```python
from build123d import *

# Parameters (mm, degrees)
BOSS_EXTRUDE1_DEPTH = 5
SKETCH11_R          = 7.25
BOSS_EXTRUDE3_DEPTH = 0.5
SKETCH12_R          = 6
BOSS_EXTRUDE4_DEPTH = 3.5
SKETCH13_R          = 1.55
CUT_EXTRUDE1_DEPTH  = 20.5
CUT_EXTRUDE2_DEPTH  = 2.6
SKETCH17_R          = 1.55
CUT_EXTRUDE4_DEPTH  = 10.02
SKETCH18_R          = 2.85
CUT_EXTRUDE5_DEPTH  = 2.85
CUT_EXTRUDE7_DEPTH  = 10


with BuildPart() as part:
    # Sketch2 → Boss-Extrude1 (new body)
    with BuildSketch(Plane.XY):
        with BuildLine():
            Line((0, 11.5), (90, 11.5))
            ThreePointArc((90, 11.5), (101.5, 0), (90, -11.5))
            Line((90, -11.5), (0, -11.5))
            ThreePointArc((0, -11.5), (-11.5, 0), (0, 11.5))
        make_face()
    extrude(amount=-BOSS_EXTRUDE1_DEPTH)

    # Sketch11 → Boss-Extrude3 (add)
    with BuildSketch(Plane.XY):
        with Locations((90, 0)):
            Circle(SKETCH11_R)
    extrude(amount=BOSS_EXTRUDE3_DEPTH)

    # Sketch12 → Boss-Extrude4 (add)
    with BuildSketch(Plane.XY.offset(0.5)):
        with Locations((90, 0)):
            Circle(SKETCH12_R)
    extrude(amount=BOSS_EXTRUDE4_DEPTH)

    # Sketch13 → Cut-Extrude1 (cut)
    with BuildSketch(Plane.XY.offset(4)):
        with Locations((90, 0)):
            Circle(SKETCH13_R)
    extrude(amount=-CUT_EXTRUDE1_DEPTH, mode=Mode.SUBTRACT)

    # Sketch14 → Cut-Extrude2 (cut)
    with BuildSketch(Plane(origin=(0, 0, -5), x_dir=(-1, 0, 0), z_dir=(0, 0, -1))):
        Polygon((-93.213605432, -0.355068252), (-91.299304589, -2.960598068), (-88.085699158, -2.605529815), (-86.786394568, 0.355068252), (-88.700695411, 2.960598068), (-91.914300842, 2.605529815), align=None)
    extrude(amount=-CUT_EXTRUDE2_DEPTH, mode=Mode.SUBTRACT)

    # Sketch17 → Cut-Extrude4 (cut)
    with BuildSketch(Plane.XY):
        with Locations((0, 7)):
            Circle(SKETCH17_R)
        with Locations((0, -7)):
            Circle(SKETCH17_R)
        with Locations((-7, 0)):
            Circle(SKETCH17_R)
        with Locations((7, 0)):
            Circle(SKETCH17_R)
    extrude(amount=-CUT_EXTRUDE4_DEPTH, mode=Mode.SUBTRACT)

    # Sketch18 → Cut-Extrude5 (cut)
    with BuildSketch(Plane.XY):
        Circle(SKETCH18_R)
    extrude(amount=-CUT_EXTRUDE5_DEPTH, mode=Mode.SUBTRACT)

    # Sketch19 → Cut-Extrude7 (cut)
    with BuildSketch(Plane.XY):
        with BuildLine():
            Line((30.521520475, -8), (15.521520475, 8))
            ThreePointArc((15.521520475, 8), (12.69309335, 6.828427125), (11.521520475, 4))
            Line((11.521520475, 4), (11.521520475, -4))
            ThreePointArc((11.521520475, -4), (12.69309335, -6.828427125), (15.521520475, -8))
            Line((15.521520475, -8), (30.521520475, -8))
        make_face()
        Polygon((50.521520475, 8), (20.521520475, 8), (35.521520475, -8), align=None)
        Polygon((70.521520475, -8), (55.521520475, 8), (40.521520475, -8), align=None)
        with BuildLine():
            Line((75.521520475, 8), (60.521520475, 8))
            Line((60.521520475, 8), (75.521520475, -8))
            ThreePointArc((75.521520475, -8), (78.3499476, -6.828427125), (79.521520475, -4))
            Line((79.521520475, -4), (79.521520475, 4))
            ThreePointArc((79.521520475, 4), (78.3499476, 6.828427125), (75.521520475, 8))
        make_face()
    extrude(amount=-CUT_EXTRUDE7_DEPTH, mode=Mode.SUBTRACT)


solid = part.part
```
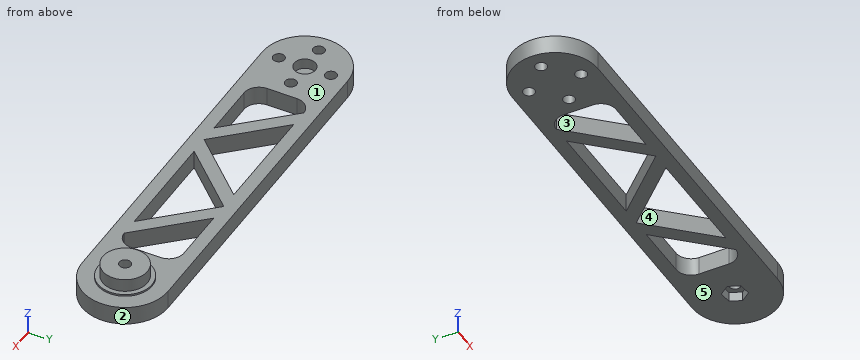
Geometry check sheet. Reference: the model listing, model coordinates, mm. Face numbers are marked on the shaded views. A direction names the side the tool comes from. Coordinates: 2 decimals unless noted, no trailing zeros. Write each loop counter-clockwise with the first axis right and the second up, starting at its lowest first coordinate (ties: lowest second). Pieces come first, ordered by that corner, then holes. Notation, with made-up numbers: (24, -15.5) -> (65, -15.5) arc R26 cw to (65, 7.5) -> close; hole circle Ø11 at (60, 70). An arc over 180 degrees is marked (long way). Use CSV: the item, a comma, the result in double quotes. Start each with the question number.
Item 1: Depth check by flat-ended pin: pin 1 Ø1.5 at (y, z) = (1, -1.5) entering from -X; pin 2 Ø4 at (x, y) = (9.5, -4.5) entering from +Z; pin 3 Ø5 at (y, z) = (-6, -1) entering from +X; pin 4 Ø6.5 at (x, y) = (91, 1) entering from -Z. Enter the tip coordinate at first touch or a pass-through.
Item 2: Cross-section at A-A, the plane x = 7. Record the cut outline in (y, z).
Item 3: Thickness scan on line 1 (Y direction, x = 0, z = -3.55); line 2 (X direction, y = -6, z = -3.75); line 3 (X direction, y = 3, z = -3.5). Record the ranges inside material, lowest first.
Item 4: Cross-section at B-B, the plane z = 1.75. Record the cut outline in (x, y).
Item 5: Set-up check for the marked faces 4 and 5: record each of +Z, -Z, +X, -X, +Y, -Y from which the full face is reachable in a straight line by a thin tool's end or side.
Item 6: Mould release check, pull along X, two halves, no side actions. Record for the marked faces 1, 2 and 3: released by +X, released by -X, zero draft, split by the parting line, or undercut.
Item 7: Cross-section at C-C, the plane x = -7. Record the cut outline in (y, z), plus the area to 3 significant figures.
Answers:
1,pin 1,"x = -11.5"
1,pin 2,"z = 0"
1,pin 3,"x = 100.95"
1,pin 4,"z = -5"
2,outline,"(-11.5, -5) -> (-1.55, -5) -> (-1.55, 0) -> (-11.5, 0) -> close; (1.55, -5) -> (11.5, -5) -> (11.5, 0) -> (1.55, 0) -> close"
3,line 1,"-11.5 to -8.55, -5.45 to 5.45, 8.55 to 11.5"
3,line 2,"-9.81 to -1.18, 1.18 to 12.06, 28.65 to 33.65, 37.4 to 42.4, 68.65 to 73.65, 78.99 to 99.81"
3,line 3,"-11.1 to 11.52, 20.21 to 25.21, 45.83 to 50.83, 60.21 to 65.21, 79.52 to 101.1"
4,outline,"circle Ø12 at (90, 0); hole circle Ø3.1 at (90, 0)"
5,face 4,"+Z, -Z"
5,face 5,"-Z, +X, -X, +Y, -Y"
6,face 1,"zero draft"
6,face 2,"released by +X"
6,face 3,"undercut"
7,outline,"(-9.12, -5) -> (-1.55, -5) -> (-1.55, 0) -> (-9.12, 0) -> close; (1.55, -5) -> (9.12, -5) -> (9.12, 0) -> (1.55, 0) -> close"
7,area,"75.7 mm^2"
